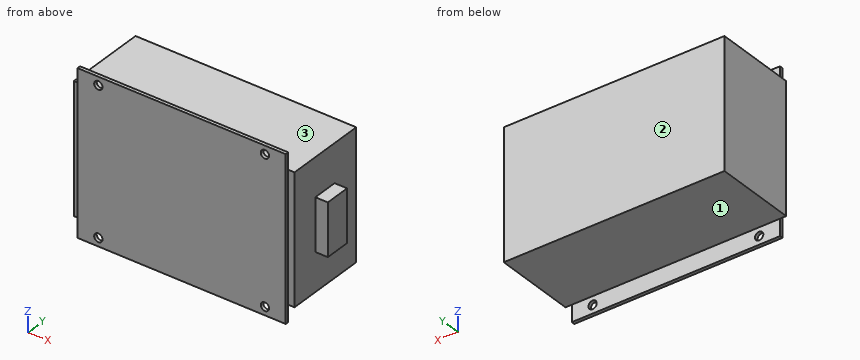
from build123d import *

# Parameters (mm, degrees)
SKETCH1_W           = 100
SKETCH1_H           = 78
SKETCH1_R           = 2
BOSS_EXTRUDE1_DEPTH = 1.5875
SKETCH2_W           = 106
SKETCH2_H           = 62
BOSS_EXTRUDE2_DEPTH = 39.4125
SKETCH3_W           = 25.156810392
SKETCH3_H           = 12.296698836
BOSS_EXTRUDE3_DEPTH = 6


with BuildPart() as part:
    # Sketch1 → Boss-Extrude1 (new body)
    with BuildSketch(Plane(origin=(0, 0, 0), x_dir=(1, 0, 0), z_dir=(0, 1, 0))):
        Rectangle(SKETCH1_W, SKETCH1_H)
        with Locations(Location((-40, 35, 0), (0, 0, 270))):
            Circle(SKETCH1_R, mode=Mode.SUBTRACT)
        with Locations(Location((40, 35, 0), (0, 0, 270))):
            Circle(SKETCH1_R, mode=Mode.SUBTRACT)
        with Locations(Location((-40, -35, 0), (0, 0, 270))):
            Circle(SKETCH1_R, mode=Mode.SUBTRACT)
        with Locations(Location((40, -35, 0), (0, 0, 270))):
            Circle(SKETCH1_R, mode=Mode.SUBTRACT)
    extrude(amount=BOSS_EXTRUDE1_DEPTH)

    # Sketch2 → Boss-Extrude2 (add)
    with BuildSketch(Plane(origin=(0, 1.5875, 0), x_dir=(-1, 0, 0), z_dir=(0, 1, 0))):
        Rectangle(SKETCH2_W, SKETCH2_H)
    extrude(amount=BOSS_EXTRUDE2_DEPTH)

    # Sketch3 → Boss-Extrude3 (add)
    with BuildSketch(Plane(origin=(53, 0, 0), x_dir=(0, 0, -1), z_dir=(1, 0, 0))):
        with Locations((0, 21.048260477)):
            Rectangle(SKETCH3_W, SKETCH3_H)
    extrude(amount=BOSS_EXTRUDE3_DEPTH)


solid = part.part
Work out the finished part from the listing and answer in its coordinate system (mm). Face numbers are marked on the shaded views. A direction names the side the tool comes from. Give positions to 0.01 mm unless a question says otherwise; leave off trailing zeros. Loops run counter-clockwise (first coordinate to the right, second up) from the corner with the lowest first, then second, coordinate; pieces in that order, holes last. Notation, with made-up numbers: (21, -5.5) -> (66, -5.5) arc R22 cw to (66, 10.5) -> close; hole circle Ø5 at (29.5, -2.75). An arc over 180 degrees is marked (long way). Use a Markdown table: item, result. Add a question column.
1) The part is cut by section C-C, the plane z = -17.5. Determine the outline of the cut face in (x, y).
2) Each of these flat-tipped pins is pushed along its axis until it touches: P1, Ø10, axis at x = 37, y = 36.5, coming from the -Z side; P2, Ø1.3, axis at y = 1, z = -17.5, coming from the +X side; P3, Ø6.5, axis at x = 40, z = 35, coming from the +Y side. Where does it stop, or does it pass through?
3) Consider line 1 along X through (y, z) = (1, -35); line 2 along Z through (x, y) = (13.5, 11); line 3 along Y through (x, z) = (44.5, 35.5). Determine where each line is inside the solid, lowest interval first.
4) The part is cut by section A-A, the plane x = 40. Determine the outline of the cut face in (y, z).
5) The part is cut by section B-B, the plane z = 35. Determine the outline of the cut face in (x, y).
6) The part is cut by section D-D, the plane x = -28. Determine the outline of the cut face in (y, z).
7) Which of the six approach directions +Z, -Z, +X, -X, +Y, -Y give full straight-line access (tool end or side, diameter ignored) to the marked faces 1, 2 and 3?
Reported:
| question | item | result |
|---|---|---|
| 1 | outline | (-53, 1.59) -> (-50, 1.59) -> (-50, 0) -> (50, 0) -> (50, 1.59) -> (53, 1.59) -> (53, 41) -> (-53, 41) -> close |
| 2 | P1 | stops at z = -31 |
| 2 | P2 | stops at x = 53 |
| 2 | P3 | stops at y = 1.59 |
| 3 | line 1 | x = -50 to -42, -38 to 38, 42 to 50 |
| 3 | line 2 | z = -31 to 31 |
| 3 | line 3 | y = 0 to 1.59 |
| 4 | outline | (0, -39) -> (1.59, -39) -> (1.59, -37) -> (0, -37) -> close; (0, -33) -> (1.59, -33) -> (1.59, -31) -> (41, -31) -> (41, 31) -> (1.59, 31) -> (1.59, 33) -> (0, 33) -> close; (0, 37) -> (1.59, 37) -> (1.59, 39) -> (0, 39) -> close |
| 5 | outline | (-50, 0) -> (-42, 0) -> (-42, 1.59) -> (-50, 1.59) -> close; (-38, 0) -> (38, 0) -> (38, 1.59) -> (-38, 1.59) -> close; (42, 0) -> (50, 0) -> (50, 1.59) -> (42, 1.59) -> close |
| 6 | outline | (0, -39) -> (1.59, -39) -> (1.59, -31) -> (41, -31) -> (41, 31) -> (1.59, 31) -> (1.59, 39) -> (0, 39) -> close |
| 7 | face 1 | -Z, +X, -X, +Y |
| 7 | face 2 | +Z, -Z, +X, -X, +Y |
| 7 | face 3 | +Z, +X, -X, +Y |
